Build history of the part. All positions in model axes, mm. A direction names the side the tool comes from. Give positions to 0.01 mm unless a question says otherwise; leave off trailing zeros. Order: outer loops, then holes, each group sorted by start corner. A loop starts at its lowest first (then second) coordinate and runs counter-clockwise, first axis right, second up. Notation, with made-up numbers: (34.5, 82) - (57.5, 82) arc R13 ccw to (57.5, 106) - close; hole circle Ø5 at (4.5, -38). An arc over 180 degrees is marked (long way). One line per item, written item: value.
Autodesk Inventor part; units mm, degrees
ref_plane "YZ Plane" through (0, 0, 0) normal (1, 0, 0) x (0, 1, 0)
ref_plane "XZ Plane" through (0, 0, 0) normal (0, 1, 0) x (-1, 0, 0)
ref_plane "XY Plane" through (0, 0, 0) normal (0, 0, 1) x (1, 0, 0)
sketch "Sketch1" plane through (0, 0, 0) normal (0, 0, 1) x (1, 0, 0)
  line L0 (0, 0) -> (12.7, 0)
  line L1 (12.7, 0) -> (12.7, 35.56)
  line L2 (12.7, 35.56) -> (0, 35.56)
  line L3 (0, 35.56) -> (0, 0)
  line L4 (1.27, 34.29) -> (11.43, 34.29)
  line L5 (11.43, 34.29) -> (11.43, 1.27)
  line L6 (11.43, 1.27) -> (1.27, 1.27)
  line L7 (1.27, 1.27) -> (1.27, 34.29)
  dimension "d0" = 35.56
  dimension "d1" = 12.7
  dimension "d2" = 1.27
extrude "Extrusion1" add sketch "Sketch1" along normal blind 127
sketch "Sketch2" plane through (12.7, 0, 0) normal (1, 0, 0) x (0, 0, -1)
  line L0 (-168.1044, 17.78) -> (-15.152, 17.78) construction
  line L1 (0, 0) -> (-127, 0) construction
  line L2 (-127, 0) -> (-127, 35.56)
  line L3 (0, 0) -> (0, 35.56)
  point P0 (-101.6, 17.78)
  point P1 (-25.4, 17.78)
  dimension "d5" = 17.78
  dimension "d6" = 25.4
  dimension "d7" = 25.4
hole "Hole1" at (12.7, 17.78, 101.6) at (12.7, 17.78, 25.4) direction (-1, 0, 0) diameter 3.2639 end through all
sketch "Sketch4" plane through (0, 35.56, 0) normal (0, 1, 0) x (1, 0, 0)
  line L0 (6.35, 23.2485) -> (6.35, -226.9955) construction
  line L1 (12.7, 0) -> (12.7, -127) construction
  line L2 (12.7, 0) -> (0, 0)
  line L3 (0, 0) -> (0, -127)
  line L4 (12.7, -127) -> (0, -127)
  line L5 (12.7, 0) -> (12.7, -127)
  point P0 (0, 0)
  point P1 (6.35, -31.75)
  point P2 (6.35, -95.25)
  dimension "d27" = 6.35
  dimension "d28" = 31.75
  dimension "d29" = 31.75
hole "Hole3" at (6.35, 35.56, 31.75) at (6.35, 35.56, 95.25) direction (0, -1, 0) diameter 3.2512 end through all
properties part number "000101"
(1) Drill centre lines: line 1 (Z direction, x = 0.4, y = 17.78); line 2 (Z direction, x = 6.35, y = 0.45); line 3 (X direction, y = 25.5, z = 87.5). Where is each one in solid material? Low to high.
Completed:
line 1: 0 to 23.77, 27.03 to 99.97, 103.23 to 127
line 2: 0 to 30.12, 33.38 to 93.62, 96.88 to 127
line 3: 0 to 1.27, 11.43 to 12.7
(2) Pull direction Z, two halves, no side cores. Call faces 1 (the face through (6.279, 0.626, 93.626)), 2 (the face through (6.279, 34.916, 30.126)), 3 (the face through (1, 19, 127)), 4 (the face through (0, 18, 63)): +Z half, -Z half, draft (parallel to the pull), parting line (faces both ways), or undercut.
Completed:
face 1: undercut
face 2: undercut
face 3: +Z half
face 4: draft
(3) Slice it at D-D, the plane z = 31.75. Give the cut face in (x, y).
Completed:
outline: (0, 0) - (4.72, 0) - (4.72, 1.27) - (1.27, 1.27) - (1.27, 34.29) - (4.72, 34.29) - (4.72, 35.56) - (0, 35.56) - close; (7.98, 0) - (12.7, 0) - (12.7, 35.56) - (7.98, 35.56) - (7.98, 34.29) - (11.43, 34.29) - (11.43, 1.27) - (7.98, 1.27) - close
(4) Slice it at C-C, the plane z = 80. Give the cut face in (x, y), and give its area (3 significant figures).
Completed:
outline: (0, 0) - (12.7, 0) - (12.7, 35.56) - (0, 35.56) - close; hole (1.27, 1.27) - (11.43, 1.27) - (11.43, 34.29) - (1.27, 34.29) - close
area: 116 mm²
(5) Pin check, flat tip, straight feed: P1, Ø2, axis at y = 17.78, z = 25.4, coming from the -X side. Stop position of the tip, or through.
Completed:
P1: through
(6) Slice it at A-A, the plane x = 6.35. Give the cut face in (y, z).
Completed:
outline: (0, 0) - (1.27, 0) - (1.27, 30.12) - (0, 30.12) - close; (0, 33.38) - (1.27, 33.38) - (1.27, 93.62) - (0, 93.62) - close; (0, 96.88) - (1.27, 96.88) - (1.27, 127) - (0, 127) - close; (34.29, 0) - (35.56, 0) - (35.56, 30.12) - (34.29, 30.12) - close; (34.29, 33.38) - (35.56, 33.38) - (35.56, 93.62) - (34.29, 93.62) - close; (34.29, 96.88) - (35.56, 96.88) - (35.56, 127) - (34.29, 127) - close
(7) Slice it at B-B, the plane y = 14. Give the cut face in (x, z), and give its area (3 significant figures).
Completed:
outline: (0, 0) - (1.27, 0) - (1.27, 127) - (0, 127) - close; (11.43, 0) - (12.7, 0) - (12.7, 127) - (11.43, 127) - close
area: 323 mm²
(8) 3-axis set-ups, long thin cutter, end or side, ignore diameter. For faces 5 (the face through (1.27, 18, 63)), 6 (the face through (12.056, 19.373, 25.754)): which of +Z, -Z, +X, -X, +Y, -Y reach the whole face in a straight line?
Completed:
face 5: +Z, -Z
face 6: +X, -X
